Source: three-view drawing plus pictorial views. Frame: mm from the lowest corner of the part. Coordinates: 2 decimals unless noted, no trailing zeros. Write each loop counter-clockwise with the first axis right and the second up, starting at its lowest first coordinate (ties: lowest second). Pieces come first, ordered by that corner, then holes. Notation, with made-up numbers: (-39.75, 6.25) - (18.25, 6.25) arc R19 cw to (18.25, 39.25) - close; hole circle Ø4 at (-21.75, -29). An arc over 180 degrees is marked (long way). Put each result on its own line as item: value. Start each with the question number.
1. Pin query (flat end, axial travel): pin 1 (1 mm diameter, centred on y = 2, z = 178.5, fed in from -X). Return the tip coordinate at first contact, or that it passes through.
2. Cut plane A-A, the plane x = 104. Return loops of the section in (y, z) (3 decimals), and give its area (3 significant figures).
3. Line query: line 1 (X direction, y = 1, z = 85.5) (3 decimals); line 2 (Z direction, x = 285, y = 1.4) (3 decimals); line 3 (X direction, y = 1.55, z = 232.5) (3 decimals). Output: solid intervals per line, ascending.
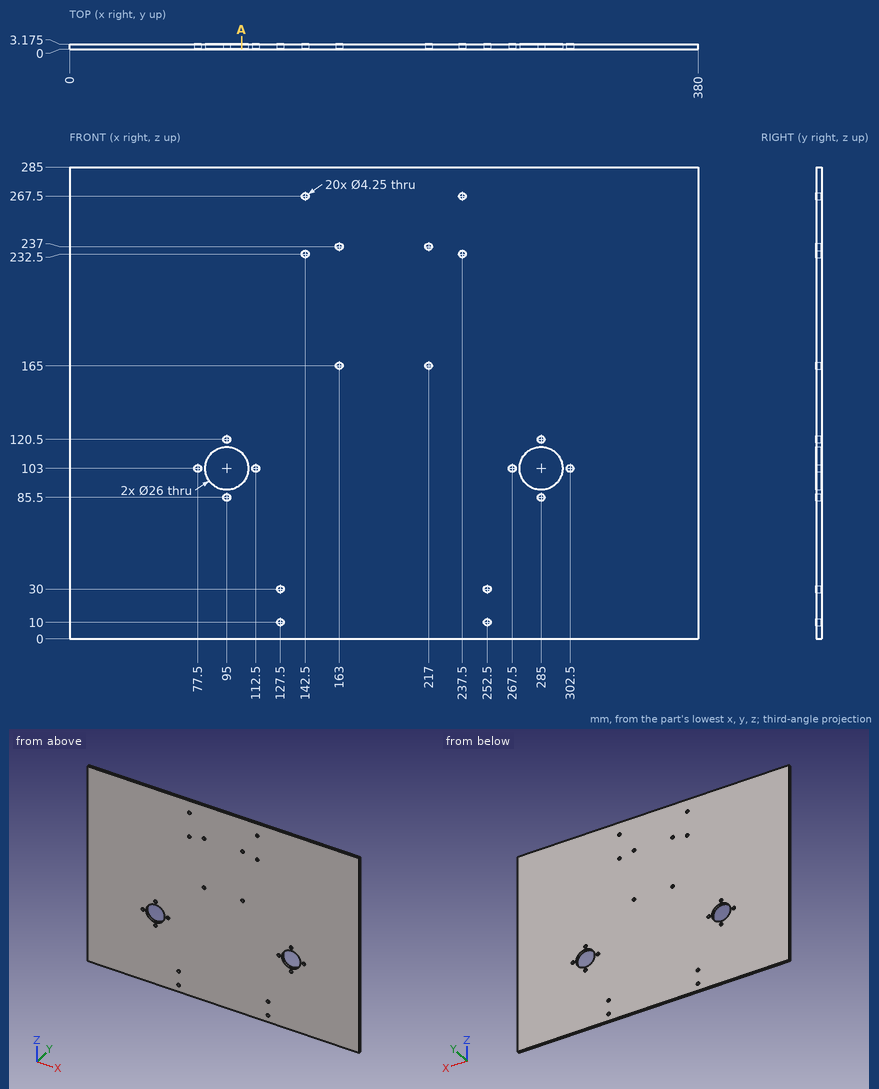
Report:
1. pin 1: stops at x = 0
2. outline: (0, 0) - (3.175, 0) - (3.175, 93.619) - (0, 93.619) - close; (0, 112.381) - (3.175, 112.381) - (3.175, 285) - (0, 285) - close
2. area: 845 mm^2
3. line 1: x = 0 to 92.875, 97.125 to 282.875, 287.125 to 380
3. line 2: z = 0 to 83.375, 87.625 to 90, 116 to 118.375, 122.625 to 285
3. line 3: x = 0 to 140.375, 144.625 to 235.375, 239.625 to 380
